```python
from build123d import *

# Parameters (mm, degrees)
F0_W     = 9
F0_H     = 9
F1_DEPTH = 42
F2_R     = 1
F3_W     = 7.2
F3_H     = 7.2
F4_DEPTH = 41
F5_R     = 0.5


with BuildPart() as f1:
    # F0 (on Top) → F1 (new body)
    with BuildSketch(Plane.XY):
        Rectangle(F0_W, F0_H)
    extrude(amount=F1_DEPTH)

    # F2
    f2_edges = [f1.edges().sort_by_distance(p)[0] for p in [
        (-4.5, -4.5, 21),
        (4.5, -4.5, 21),
        (4.5, 4.5, 21),
        (-4.5, 4.5, 21),
    ]]
    fillet(f2_edges, radius=F2_R)

    # F3 (on face) → F4 (cut)
    with BuildSketch(Plane.XY.offset(42)):
        Rectangle(F3_W, F3_H)
    extrude(amount=-F4_DEPTH, mode=Mode.SUBTRACT)

    # F5
    f5_edges = [f1.edges().sort_by_distance(p)[0] for p in [
        (0, 3.6, 1),
        (-3.6, 0, 1),
        (3.6, 0, 1),
        (0, -3.6, 1),
    ]]
    fillet(f5_edges, radius=F5_R)


solid = f1.part
```
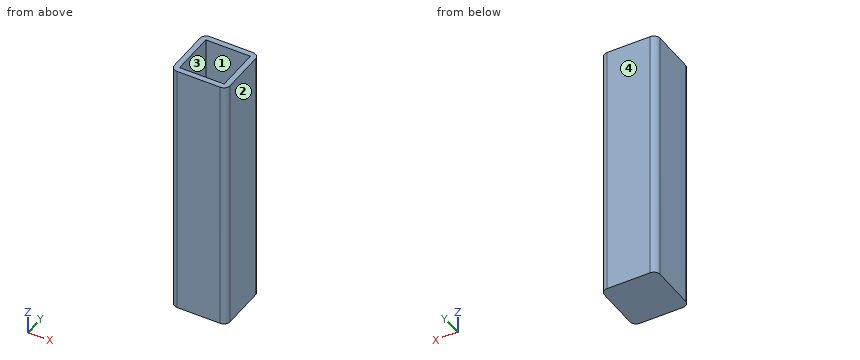
Can you work these out from the model? Positions are in its coordinate system, mm. Face numbers are marked on the shaded views. Coordinates: 2 decimals unless noted, no trailing zeros. Write each loop counter-clockwise with the first axis right and the second up, starting at its lowest first coordinate (ties: lowest second). Pieces come first, ordered by that corner, then holes. Notation, with made-up numbers: M 73,15 L 100,15 A31 cw 100,40 Z; hole C 56.25,6.25 d10. An arc over 180 degrees is marked long. Answer as CSV lines item,"result".
Item 1: We'd pull the mould along X, two halves only. Please class the marked faces 1, 2, 3 and 4: +X half, -X half, draft (parallel to the pull), parting line (faces both ways), or undercut.
Geometry results:
face 1,"undercut"
face 2,"+X half"
face 3,"undercut"
face 4,"draft"
Item 2: Please list where these lines run through material, in increasing order: line 1 along Y through (x, z) = (2.75, 23); line 2 along Z through (x, y) = (-1, -2).
Geometry results:
line 1,"y = -4.5 to -3.6, 3.6 to 4.5"
line 2,"z = 0 to 1"
Item 3: I'm going to push flat-ended pins straight in: P1, Ø5, axis at x = -0.5, y = 0, coming from the +Z side; P2, Ø2, axis at x = 0.5, y = -3.5, coming from the +Z side. Where does each tip first touch, or does it pass through?
Geometry results:
P1,"stops at z = 1"
P2,"stops at z = 42"
Item 4: Imagine slicing it at B-B on x = 1.5. List the corners of the cut face in (y, z) for me, plus the area to 3 significant figures.
Geometry results:
outline,"M -4.5,0 L 4.5,0 L 4.5,42 L 3.6,42 L 3.6,1.5 A0.5 cw 3.1,1 L -3.1,1 A0.5 cw -3.6,1.5 L -3.6,42 L -4.5,42 Z"
area,"82.9 mm2"
Item 5: Imagine slicing it at A-A on z = 38. List the corners of the cut face in (x, y) for me, plus the area to 3 significant figures.
Geometry results:
outline,"M -4.5,-3.5 A1 ccw -3.5,-4.5 L 3.5,-4.5 A1 ccw 4.5,-3.5 L 4.5,3.5 A1 ccw 3.5,4.5 L -3.5,4.5 A1 ccw -4.5,3.5 Z; hole M -3.6,-3.6 L 3.6,-3.6 L 3.6,3.6 L -3.6,3.6 Z"
area,"28.3 mm2"
